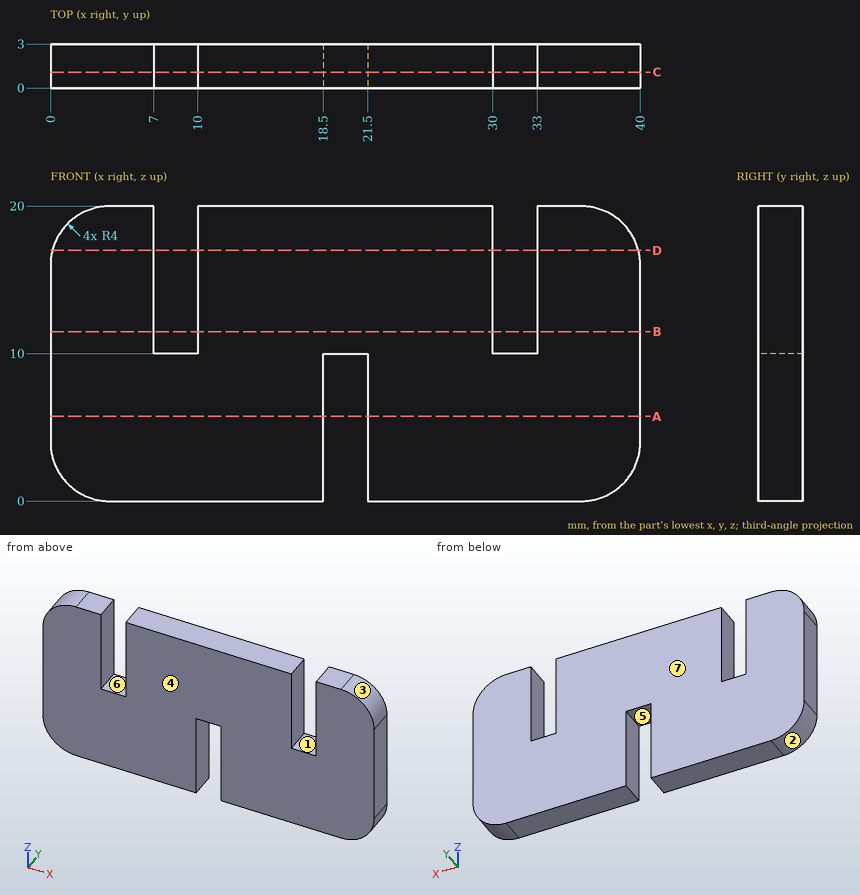
Design review of the part shown in the three views and the two pictorial views. Dimensions are in mm from the part's minimum x, y and z. A direction names the side the tool comes from. Round coordinates to 2 decimals unless told otherwise and drop trailing zeros. Write each loop counter-clockwise with the first axis right and the second up, starting at its lowest first coordinate (ties: lowest second). Pieces come first, ordered by that corner, then holes. Notation, with made-up numbers: M -2.5,47 L 41.5,47 A24 cw 41.5,66 Z; hole C -1,65 d2. An arc over 180 degrees is marked long. One line per item, written item: value. Start each with the question number.
1. For the marked faces 5, 6 and 7, list the 3-axis set-ups (+Z, -Z, +X, -X, +Y, -Y) from which the entire face can be reached by the end or side of a thin tool; tool diameter is ignored.
2. Take a section at D-D on z = 17. State the section outline as (x, y) points.
3. Take a section at B-B on z = 11.5. State the section outline as (x, y) points.
4. Draft analysis for pull direction X (two halves, no side actions). For the marked faces 1, 2, 3 and 4, state which applies: pulls with the +X half, pulls with the -X half, needs draft (parallel to the pull), parting line crosses it, or undercut.
5. Take a section at A-A on z = 5.75. State the section outline as (x, y) points.
6. Clearance check with a flat-ended pin moving along its axis: P1, Ø0.9, axis at x = 8.5, y = 2, coming from the +Z side. State where the tip first meets the part, or that it passes through.
7. Take a section at C-C on y = 1.1. State the section outline as (x, z) points.
8. To check wall thickness, follow probe 1 along X at (y, z) = (0.3, 11.25); probe 2 along X at (y, z) = (2.25, 6.75); probe 3 along X at (y, z) = (2.7, 19.25). State the ranges of each line that lie inside material, in increasing order. Write a range as from..to.
Computed:
1. face 5: -Z, +Y, -Y
1. face 6: +Z, +Y, -Y
1. face 7: +Z, -Z, +X, -X, +Y
2. outline: M 0.13,0 L 7,0 L 7,3 L 0.13,3 Z; M 10,0 L 30,0 L 30,3 L 10,3 Z; M 33,0 L 39.87,0 L 39.87,3 L 33,3 Z
3. outline: M 0,0 L 7,0 L 7,3 L 0,3 Z; M 10,0 L 30,0 L 30,3 L 10,3 Z; M 33,0 L 40,0 L 40,3 L 33,3 Z
4. face 1: undercut
4. face 2: pulls with the -X half
4. face 3: pulls with the +X half
4. face 4: needs draft
5. outline: M 0,0 L 18.5,0 L 18.5,3 L 0,3 Z; M 21.5,0 L 40,0 L 40,3 L 21.5,3 Z
6. P1: stops at z = 10
7. outline: M 0,4 A4 ccw 4,0 L 18.5,0 L 18.5,10 L 21.5,10 L 21.5,0 L 36,0 A4 ccw 40,4 L 40,16 A4 ccw 36,20 L 33,20 L 33,10 L 30,10 L 30,20 L 10,20 L 10,10 L 7,10 L 7,20 L 4,20 A4 ccw 0,16 Z
8. probe 1: x = 0..7, 10..30, 33..40
8. probe 2: x = 0..18.5, 21.5..40
8. probe 3: x = 1.67..7, 10..30, 33..38.33
